The listing builds one solid part. Answer for the finished solid, in the listing's coordinates (mm). Coordinates: 2 decimals unless noted, no trailing zeros. Order: outer loops, then holes, each group sorted by start corner. A loop starts at its lowest first (then second) coordinate and runs counter-clockwise, first axis right, second up.
from build123d import *

# Parameters (mm, degrees)
SKETCH_R  = 1.8288
PAD_DEPTH = 3


with BuildPart() as part:
    # Sketch → Pad (new body)
    with BuildSketch(Plane.XY):
        with BuildLine():
            ThreePointArc((5.800476, 50.8), (5.263177, 50.643391), (4.894168, 50.222618))
            Line((4.894168, 50.222618), (-30.1, -24.822618))
            ThreePointArc((-31.006308, -25.4), (-30.469008, -25.243391), (-30.1, -24.822618))
            Line((-37.1, -25.4), (-31.006308, -25.4))
            ThreePointArc((-37.1, -25.4), (-37.807107, -25.692893), (-38.1, -26.4))
            Line((-38.1, -49.8), (-38.1, -26.4))
            ThreePointArc((-38.1, -49.8), (-37.807107, -50.507107), (-37.1, -50.8))
            Line((-37.1, -50.8), (-23.352, -50.8))
            ThreePointArc((-23.352, -50.8), (-22.644893, -50.507107), (-22.352, -49.8))
            Line((-22.352, -38.1), (-22.352, -49.8))
            ThreePointArc((-15.748, -38.1), (-19.05, -34.798), (-22.352, -38.1))
            Line((-15.748, -38.1), (-15.748, -49.8))
            ThreePointArc((-15.748, -49.8), (-15.455107, -50.507107), (-14.748, -50.8))
            Line((-14.748, -50.8), (14.748, -50.8))
            ThreePointArc((14.748, -50.8), (15.455107, -50.507107), (15.748, -49.8))
            Line((15.748, -38.1), (15.748, -49.8))
            ThreePointArc((22.352, -38.1), (19.05, -34.798), (15.748, -38.1))
            Line((22.352, -38.1), (22.352, -49.8))
            ThreePointArc((22.352, -49.8), (22.644893, -50.507107), (23.352, -50.8))
            Line((23.352, -50.8), (37.1, -50.8))
            ThreePointArc((37.1, -50.8), (37.807107, -50.507107), (38.1, -49.8))
            Line((38.1, 49.8), (38.1, -49.8))
            ThreePointArc((38.1, 49.8), (37.807107, 50.507107), (37.1, 50.8))
            Line((5.800476, 50.8), (37.1, 50.8))
        make_face()
        with Locations((24.6352, 44.45)):
            Circle(SKETCH_R, mode=Mode.SUBTRACT)
    extrude(amount=PAD_DEPTH)


solid = part.part
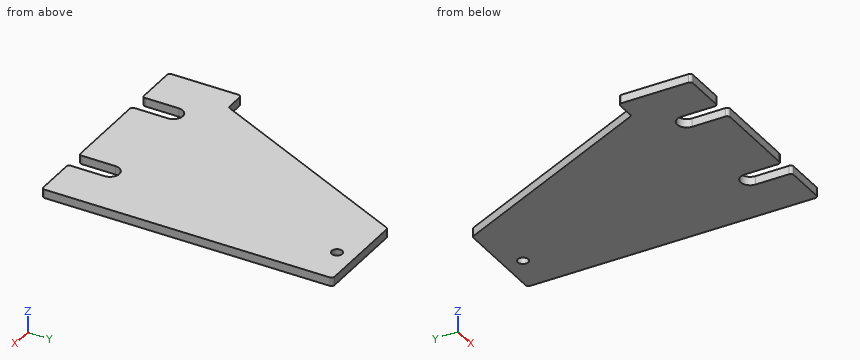
1) Section D-D (y = 34) is taken. Give the vertices of the cut face in (x, z).
2) Consider L1, parallel to X at y = -39.5, z = 2.95; L2, parallel to Y at x = -31, z = 1.1; L3, parallel to X at y = -10, z = 1.45. Determine where each line is inside the solid, lowest interval first.
3) This flat-tipped pin is pushed along its axis until it touches: P1, Ø10, axis at x = 3, y = -19.5, coming from the -Z side. Where does it stop, or does it pass through?
4) Section C-C (x = -28) is taken. Give the vertices of the cut face in (y, z).
5) Section B-B (y = 44.45) is taken. Give the vertices of the cut face in (x, z), then the cut area to 3 significant figures.
6) Section A-A (z = 2.3) is taken. Give the vertices of the cut face in (x, y).
Filled sheet:
1. outline: (-2.67, 0) - (38.1, 0) - (38.1, 3) - (-2.67, 3) - close
2. L1: x = -38.1 to -22.35, -15.75 to 15.75, 22.35 to 38.1
2. L2: y = -50.8 to -25.4
2. L3: x = -23.19 to 38.1
3. P1: stops at z = 0
4. outline: (-50.8, 0) - (-20.32, 0) - (-20.32, 3) - (-50.8, 3) - close
5. outline: (2.2, 0) - (22.81, 0) - (22.81, 3) - (2.2, 3) - close; (26.46, 0) - (38.1, 0) - (38.1, 3) - (26.46, 3) - close
5. area: 96.7 mm2
6. outline: (-38.1, -49.8) arc R1 ccw to (-37.1, -50.8) - (-23.35, -50.8) arc R1 ccw to (-22.35, -49.8) - (-22.35, -38.1) arc R3.3 cw to (-15.75, -38.1) - (-15.75, -49.8) arc R1 ccw to (-14.75, -50.8) - (14.75, -50.8) arc R1 ccw to (15.75, -49.8) - (15.75, -38.1) arc R3.3 cw to (22.35, -38.1) - (22.35, -49.8) arc R1 ccw to (23.35, -50.8) - (37.1, -50.8) arc R1 ccw to (38.1, -49.8) - (38.1, 49.8) arc R1 ccw to (37.1, 50.8) - (5.8, 50.8) arc R1 ccw to (4.89, 50.22) - (-30.1, -24.82) arc R1 cw to (-31.01, -25.4) - (-37.1, -25.4) arc R1 ccw to (-38.1, -26.4) - close; hole circle Ø3.66 at (24.64, 44.45)
